Input: part model. Units: mm. Frame: model coordinates. A direction names the side the tool comes from. Give positions to 0.01 mm unless a question says otherwise; leave off trailing zeros. Order: outer loops, then holes, each group sorted by start corner. A loop starts at its lowest first (then second) coordinate and runs counter-clockwise, first axis right, second up. Notation, with made-up numbers: (74.25, 51.25) -> (81.25, 51.25) arc R6 ccw to (81.25, 61.25) -> close; hole circle Ø11 at (-6, 83.25). An arc over 180 degrees is marked (long way). Use a Markdown table: item, result. Add a question column.
Autodesk Inventor part; units mm, degrees
ref_plane "IP_1_BO_XY" through (0, 24, 0) normal (1, 0, 0) x (0, 0, -1)
ref_plane "IP_1_BO_YZ" through (0, 24, 0) normal (0, 0, -1) x (0, 1, 0)
ref_plane "IP_1_BO_ZX" through (0, 24, 0) normal (0, 1, 0) x (1, 0, 0)
sketch "Sketch_4" plane through (0, 0, 0) normal (0, 0, 1) x (1, 0, 0)
  line L0 (0, -36) -> (0, 41)
  arc A0 (17, 24) -> (0, 41) centre (0, 24) ccw
  arc A1 (7.5441, 3.1836) -> (17, 24) centre (-8.9892, 23.2497) ccw
  arc A2 (7.5441, 3.1836) -> (7, 1.1694) centre (11, 1.1694) ccw
  line L1 (7, 1.1694) -> (7, -33.5751)
  line L2 (7, -33.5751) -> (5.6, -36)
  line L3 (5.6, -36) -> (0, -36)
  line L4 (0, -36) -> (0, 41)
revolve "Revolution1" add sketch "Sketch_4" angle 360 about axis through (0, -36, 0) along (0, -1, 0)
thread "Thread1"
sketch "Sketch_5" plane through (0, 0, 0) normal (0, 0, 1) x (1, 0, 0)
  line L0 (-25.5, 42.8) -> (-25.5, -39.6)
  line L1 (-25.5, -39.6) -> (25.5, -39.6)
  line L2 (25.5, -39.6) -> (25.5, 42.8)
  line L3 (25.5, 42.8) -> (-25.5, 42.8)
  line L4 (-7, 2.25) -> (-7, -36)
  line L5 (-7, -36) -> (7, -36)
  line L6 (7, -36) -> (7, 2.25)
  line L7 (7, 2.25) -> (3.7501, 5.5)
  line L8 (3.7501, 5.5) -> (3.7501, 41)
  line L9 (3.7501, 41) -> (-3.7501, 41)
  line L10 (-3.7501, 41) -> (-3.7501, 5.5)
  line L11 (-3.7501, 5.5) -> (-7, 2.25)
extrude "Extrusion1" cut sketch "Sketch_5" along normal mid plane 34
sketch "Sketch_6" plane through (0, 0, 0) normal (0, 0, 1) x (1, 0, 0)
  line L0 (6.75, 24) -> (-6.75, 24)
  line L1 (-6.75, 24) -> (-6.75, 38.053)
  arc A0 (-3.7501, 39.6) -> (-6.75, 38.053) centre (2.3958, 24.0001) ccw
  line L2 (-3.7501, 39.6) -> (3.7501, 39.6)
  arc A1 (6.75, 38.053) -> (3.7501, 39.6) centre (-2.3958, 24.0001) ccw
  line L3 (6.75, 38.053) -> (6.75, 24)
  line L4 (6.75, 24) -> (-6.75, 24)
revolve "Revolution2" add sketch "Sketch_6" angle 360 about axis through (6.75, 24, 0) along (1, 0, 0)
sketch "Sketch_7" plane through (0, 0, 0) normal (0, 0, 1) x (1, 0, 0)
  line L0 (12.7, 24) -> (-12.7, 24)
  arc A0 (12.7, 24) -> (-12.7, 24) centre (0, 24) ccw
  line L1 (12.7, 24) -> (-12.7, 24)
revolve "Revolution3" cut sketch "Sketch_7" angle 360 about axis through (12.7, 24, 0) along (1, 0, 0)
ref_plane "IP_1_BO_XY" through (0, 24, 0) normal (1, 0, 0) x (0, 0, -1)
ref_plane "IP_1_BO_YZ" through (0, 24, 0) normal (0, 0, -1) x (0, 1, 0)
ref_plane "IP_1_BO_ZX" through (0, 24, 0) normal (0, 1, 0) x (1, 0, 0)
properties part number "POS 14ECBody"
Q1. Draft query along Y for faces 1 (the flat face through (-4.99, 4.26, -0.13)), 2 (the flat face through (3.75, 8.666, 3.61)), 3 (the flat face through (0, -36, 0)), 4 (the cylindrical face through (6.466, -16.446, -2.681)). Return one class per face: +Y half, -Y half, draft (parallel to the pull), parting line (faces both ways), or undercut.
Q2. Access query for faces 5 (the flat face through (-3.75, 8, 0)), 6 (the flat face through (6.75, 31.2, -8.3)), 7 (the flat face through (-6.75, 31.2, -8.3)), 8 (the flat face through (5.04, 4.21, -0.13)), 9 (the conical face through (5.425, -35.848, -1.708)). Directions: +Z, -Z, +X, -X, +Y, -Y. A direction counts if a zero-diameter tool reaches every point of the face in a straight line with its end or side. Return the directions, or none.
Q3. Section query A-A (x = -4.5). Give the number of separate pieces and of enclosed holes in the cut face, plus the area to 3 significant figures.
Q4. Section query B-B (y = -17.5). Return loops of the section in (x, z).
Q5. Ray query, line 1 (Y direction, x = 5.25, z = 3.5); line 2 (Y direction, x = -4.5, z = -6.5); line 3 (Y direction, x = -0.25, z = -11.5). Return the intervals inside material, ascending.
Q6. First-contact query: pin 1 (5 mm diameter, centred on x = 1, y = -10.5, fed in from -Z); pin 2 (10 mm diameter, centred on y = 3, z = -1.5, fed in from +X); pin 3 (4 mm diameter, centred on x = -2.5, y = 10, fed in from +Z); pin 4 (1.5 mm diameter, centred on y = -14.5, z = 2, fed in from +X). Flat tips, straight axial feed; report the tip coordinate or a pass-through.
Solution:
| question | item | result |
|---|---|---|
| 1 | face 1 | undercut |
| 1 | face 2 | undercut |
| 1 | face 3 | -Y half |
| 1 | face 4 | draft |
| 2 | face 5 | -X |
| 2 | face 6 | +Z, -Z, +X, +Y |
| 2 | face 7 | +Z, -Z, -X, +Y |
| 2 | face 8 | +Z, -Z, +X |
| 2 | face 9 | -Y |
| 3 | separate pieces | 2 |
| 3 | enclosed holes | 1 |
| 3 | area | 729 mm² |
| 4 | outline | circle Ø14 at (0, 0) |
| 5 | line 1 | y = -34.77 to 4, 9.49 to 12.98, 35.02 to 38.51 |
| 5 | line 2 | y = 3.49 to 4.75, 10.17 to 14.06, 33.94 to 37.83 |
| 5 | line 3 | y = 7.25 to 18.62, 29.38 to 36.52 |
| 6 | pin 1 | stops at z = -7 |
| 6 | pin 2 | stops at x = 7 |
| 6 | pin 3 | stops at z = 14.28 |
| 6 | pin 4 | stops at x = 6.89 |
